Check sheet for the modelled part. Datum: model origin and axes. Units: mm. Face numbers are marked on the shaded views. A direction names the side the tool comes from. Give positions to 0.01 mm unless a question says otherwise; leave off trailing zeros. Write each loop counter-clockwise with the first axis right and the second up, starting at its lowest first coordinate (ties: lowest second). Pieces come first, ordered by that corner, then holes. Notation, with made-up numbers: M -37,-23.75 L -16,-23.75 A19 cw -16,-2.75 Z; hole C -26.5,22 d7. An arc over 180 degrees is marked long. Write each question's results on one line, items separated by ' | '. Start each with the question number.
from build123d import *

# Parameters (mm, degrees)
F0_W     = 100.33
F0_H     = 137.16
F0_W_2   = 330.2
F0_H_2   = 304.8
F0_W_3   = 152.4
F0_H_3   = 152.4
F1_DEPTH = 254
F4_DEPTH = 6.35
F6_DEPTH = 6.35


with BuildPart() as f1:
    # F0 (on Top) → F1 (new body)
    with BuildSketch(Plane.XY):
        Polygon((460.5475887705, 383.838060368), (-405.5924112295, 383.838060368), (-405.5924112295, 40.938060368), (-405.5924112295, -486.111939632), (-202.3924112295, -486.111939632), (-202.3924112295, -568.661939632), (26.2075887705, -568.661939632), (172.2575887705, -568.661939632), (172.2575887705, -613.111939632), (460.5475887705, -613.111939632), (460.5475887705, -282.911939632), align=None)
        with Locations((-252.5574112295, -213.061939632)):
            Rectangle(F0_W, F0_H, mode=Mode.SUBTRACT)
        with Locations((-221.4424112295, 212.388060368)):
            Rectangle(F0_W_2, F0_H_2, mode=Mode.SUBTRACT)
        Polygon((-386.5424112295, -467.061939632), (-386.5424112295, 40.938060368), (-48.7224112295, 40.938060368), (-48.7224112295, 204.768060368), (103.6775887705, 204.768060368), (103.6775887705, 40.938060368), (281.4775887705, 40.938060368), (289.0975887705, 40.938060368), (441.4975887705, 40.938060368), (441.4975887705, -86.061939632), (441.4975887705, -93.681939632), (441.4975887705, -263.861939632), (441.4975887705, -594.061939632), (191.3075887705, -594.061939632), (191.3075887705, -263.861939632), (172.2575887705, -263.861939632), (172.2575887705, -549.611939632), (-183.3424112295, -549.611939632), (-183.3424112295, -486.111939632), (-183.3424112295, -136.861939632), (-310.3424112295, -136.861939632), (-310.3424112295, -289.261939632), (-202.3924112295, -289.261939632), (-202.3924112295, -467.061939632), align=None, mode=Mode.SUBTRACT)
        with Locations((27.4775887705, 288.588060368)):
            Rectangle(F0_W_3, F0_H_3, mode=Mode.SUBTRACT)
        with Locations((276.3975887705, 212.388060368)):
            Rectangle(F0_W_2, F0_H_2, mode=Mode.SUBTRACT)
    extrude(amount=F1_DEPTH)

    # F3 (on offset) → F4 (join)
    with BuildSketch(Plane.XY.offset(203.2)):
        Polygon((-202.2046655178, -572.2870230675), (-202.2046655178, -484.5494627953), (-481.6046655178, -484.5494627953), (-481.6046655178, -885.6354951859), (26.3953344822, -885.6354951859), (26.3953344822, -572.2870230675), align=None)
    extrude(amount=-F4_DEPTH)

    # F5 (on face) → F6 (join)
    with BuildSketch(Plane.XY.offset(203.2)):
        Polygon((-484.4706356525, 264.8289501667), (-481.6046655178, -484.5494627953), (-405.5924112295, -484.5494627953), (-405.5924112295, -486.111939632), (-401.7352461815, 264.8289501667), align=None)
    extrude(amount=-F6_DEPTH)


solid = f1.part
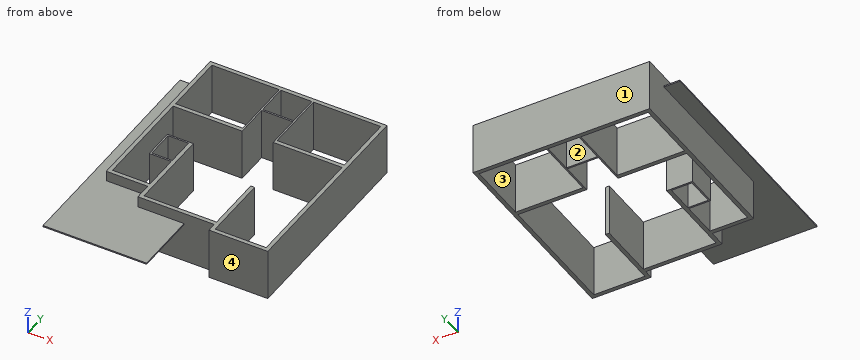
Q1. Release check for a two-part mould opening along X. For the marked faces 3 and 4 record: pulls with the +X half, pulls with the -X half, needs draft (parallel to the pull), parting line crosses it, or undercut.
Q2. Section check C-C on y = 120. Record the boundary of the cut face in (x, z).
Q3. Depth check by flat-ended pin: pin 1 Ø3 at (x, y) = (-377, -583) entering from -Z. Enter the tip coordinate at first touch or a pass-through.
Q4. Section check D-D on y = -687. Record the boundary of the cut face in (x, z), plus the area to 3 significant figures.
Q5. Scan lines: L1, parallel to Y at x = 170, z = 121.5; L2, parallel to X at y = 107, z = 132.5; L3, parallel to X at y = -163, z = 48.5. Record each from-to range of solid material in increasing order.
Q6. Tool access check on the marked faces 1 and 2. Record the directions out of +Z, -Z, +X, -X, +Y, -Y that give a thin tool (end or side, any length) a straight path to the whole face; none if there is none.
Q7. Section check B-B on z = 96. State how many separate pieces and enclosed holes the cut face has, plus the area to 3 significant figures.
Q8. Section check A-A on y = 286.5. Record the boundary of the cut face in (x, z), plus the area to 3 significant figures.
Check result:
1) face 3: undercut | face 4: needs draft
2) outline: M -483.92,196.85 L -405.59,196.85 L -405.59,0 L -386.54,0 L -386.54,254 L -405.59,254 L -405.59,203.2 L -483.92,203.2 Z; M -56.34,0 L -48.72,0 L -48.72,254 L -56.34,254 Z; M 103.68,0 L 111.3,0 L 111.3,254 L 103.68,254 Z; M 441.5,0 L 460.55,0 L 460.55,254 L 441.5,254 Z
3) pin 1: z = 196.85
4) outline: M -481.6,196.85 L 26.4,196.85 L 26.4,203.2 L -481.6,203.2 Z | area: 3,230 mm^2
5) L1: -568.66 to -549.61, 40.94 to 59.99, 364.79 to 383.84 | L2: -405.59 to -386.54, -56.34 to -48.72, 103.68 to 111.3, 441.5 to 460.55 | L3: -405.59 to -386.54, -310.34 to -302.72, -202.39 to -183.34, 441.5 to 460.55
6) face 1: +Z, -Z, +X, -X, +Y | face 2: +Z, -Z
7) separate pieces: 1 | enclosed holes: 5 | area: 103,000 mm^2
8) outline: M -405.59,0 L -386.54,0 L -386.54,254 L -405.59,254 Z; M -56.34,0 L -48.72,0 L -48.72,254 L -56.34,254 Z; M 103.68,0 L 111.3,0 L 111.3,254 L 103.68,254 Z; M 441.5,0 L 460.55,0 L 460.55,254 L 441.5,254 Z | area: 13,500 mm^2
